```python
from build123d import *

# Parameters (mm, degrees)
F0_W     = 10
F0_H     = 15
F0_H_2   = 10
F1_DEPTH = 12
F2_R     = 3
F3_DEPTH = 10.001
F4_R     = 5
F4_R_2   = 3
F5_DEPTH = 4
F6_R     = 5
F6_R_2   = 3
F7_DEPTH = 4


with BuildPart() as f1:
    # F0 (on Front) → F1 (new body)
    with BuildSketch(Plane.XZ):
        with Locations((-15, 12.5)):
            Rectangle(F0_W, F0_H)
        with Locations((-15, 0)):
            Rectangle(F0_W, F0_H_2)
        with Locations((-15, -12.5)):
            Rectangle(F0_W, F0_H)
        with BuildLine():
            Line((-10, -5), (20, -5))
            Line((20, -5), (20, 5))
            Line((20, 5), (15, 5))
            ThreePointArc((15, 5), (10, 0), (5, 5))
            Line((5, 5), (-10, 5))
            Line((-10, 5), (-10, -5))
        make_face()
    extrude(amount=F1_DEPTH)

    # F2 (on face) → F3 (cut, through all)
    with BuildSketch(Plane.YZ.offset(-10)):
        with Locations((-6, 12.5)):
            Circle(F2_R)
        with Locations((-6, -12.5)):
            Circle(F2_R)
    extrude(amount=-F3_DEPTH, mode=Mode.SUBTRACT)

    # F4 (on face) → F5 (cut)
    with BuildSketch(Plane.YZ.offset(-10)):
        with Locations((-6, 12.5)):
            Circle(F4_R)
        with Locations((-6, 12.5)):
            Circle(F4_R_2, mode=Mode.SUBTRACT)
    extrude(amount=-F5_DEPTH, mode=Mode.SUBTRACT)

    # F6 (on face) → F7 (cut)
    with BuildSketch(Plane.YZ.offset(-10)):
        with Locations((-6, -12.5)):
            Circle(F6_R)
        with Locations((-6, -12.5)):
            Circle(F6_R_2, mode=Mode.SUBTRACT)
    extrude(amount=-F7_DEPTH, mode=Mode.SUBTRACT)


solid = f1.part
```
CAD build for the part. Positions are in the model's coordinates, mm. A direction names the side the tool comes from. Round coordinates to 2 decimals unless told otherwise and drop trailing zeros. Write each loop counter-clockwise with the first axis right and the second up, starting at its lowest first coordinate (ties: lowest second). Pieces come first, ordered by that corner, then holes. Notation, with made-up numbers: (52, -16.75) - (57, -16.75) arc R7 cw to (57, -9.75) - close; hole circle Ø7 at (-19.5, 41). An arc over 180 degrees is marked (long way). Write item = value, one per line. Start each with the question number.
Q1. Which spindle directions (+Z, -Z, +X, -X, +Y, -Y) get a long thin tool onto all of the face, cutting with end or side? Do faces 5 (the flat face through (18, -6, 5)), 6 (the flat face through (-20, -6, 0)), 7 (the flat face through (-14, -4, 10)), 8 (the flat face through (5, -6, -5)). Say none if no direction does.
Q2. Band-saw the part on C-C (x = -11). Give the cut face in (y, z), then the cut area to 3 significant figures.
Q3. Mould opens along Y. For faces 1 (the flat face through (-5, 0, 0)), 2 (the flat face through (-15, -6, -20)), 3 (the cylindrical face through (-16.96, -3.14, 13.4)), 4 (the flat face through (-5, -12, 0)) say: pulls with the +Y half, pulls with the -Y half, needs draft (parallel to the pull), parting line crosses it, or undercut.
Q4. Band-saw the part on B-B (y = -6). Give the cut face in (x, z).
Q5. Drop flat-ended pins along their axis: pin 1 (6 mm diameter, centred on x = 1.5, y = -1.5, fed in from +Z); pin 2 (2 mm diameter, centred on x = -9.5, y = -6, fed in from +Z); pin 3 (6 mm diameter, centred on y = -6, z = 15, fed in from +X); pin 4 (3 mm diameter, centred on y = -6.5, z = -10, fed in from +X). Give the stop position or say it passes through.
Q6. Band-saw the part on A-A (z = 12.5). Give the cut face in (x, y), then the cut area to 3 significant figures.
Q7. Probe L1, parallel to Z at x = -17.5, y = -6; L2, parallel to Z at x = -11.55, y = -6; L3, parallel to Z at x = 15.5, y = -1.5. List the from-to ranges inside material, lowest first. Write a range as from..to.
Q8. Band-saw the part on D-D (y = -10.5). Give the cut face in (x, z).
Answers below:
q1.face_5 = +Z, +X, +Y, -Y
q1.face_6 = +Z, -Z, -X, +Y, -Y
q1.face_7 = +X
q1.face_8 = -Z, +X, +Y, -Y
q2.outline = (-12, -20) - (0, -20) - (0, 20) - (-12, 20) - close; hole circle Ø10 at (-6, -12.5); hole circle Ø10 at (-6, 12.5)
q2.area = 323 mm2
q3.face_1 = pulls with the +Y half
q3.face_2 = needs draft
q3.face_3 = undercut
q3.face_4 = pulls with the -Y half
q4.outline = (-20, -20) - (-10, -20) - (-10, -17.5) - (-14, -17.5) - (-14, -15.5) - (-20, -15.5) - close; (-20, -9.5) - (-14, -9.5) - (-14, -7.5) - (-10, -7.5) - (-10, -5) - (20, -5) - (20, 5) - (15, 5) arc R5 cw to (5, 5) - (-10, 5) - (-10, 7.5) - (-14, 7.5) - (-14, 9.5) - (-20, 9.5) - close; (-20, 15.5) - (-14, 15.5) - (-14, 17.5) - (-10, 17.5) - (-10, 20) - (-20, 20) - close
q5.pin_1 = 5
q5.pin_2 = 20
q5.pin_3 = -10
q5.pin_4 = -14
q6.outline = (-20, -12) - (-10, -12) - (-10, -11) - (-14, -11) - (-14, -9) - (-20, -9) - close; (-20, -3) - (-14, -3) - (-14, -1) - (-10, -1) - (-10, 0) - (-20, 0) - close
q6.area = 44.0 mm2
q7.L1 = -20..-15.5, -9.5..9.5, 15.5..20
q7.L2 = -20..-17.5, -7.5..7.5, 17.5..20
q7.L3 = -5..5
q8.outline = (-20, -20) - (-10, -20) - (-10, -14.68) - (-14, -14.68) - (-14, -10.32) - (-10, -10.32) - (-10, -5) - (20, -5) - (20, 5) - (15, 5) arc R5 cw to (5, 5) - (-10, 5) - (-10, 10.32) - (-14, 10.32) - (-14, 14.68) - (-10, 14.68) - (-10, 20) - (-20, 20) - close
